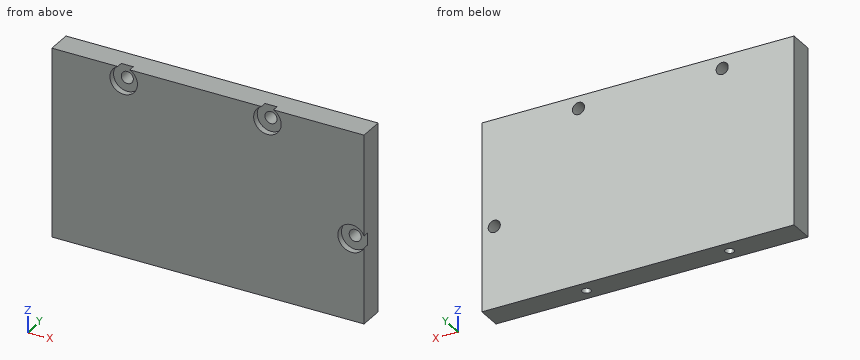
from build123d import *

# Parameters (mm, degrees)
SKETCH1_W                                           = 63
SKETCH1_H                                           = 38
BOSS_EXTRUDE1_DEPTH                                 = 5
CBORE_FOR_2_BINDING_HEAD_MACHINE_SCREW2_D           = 2.4384
CBORE_FOR_2_BINDING_HEAD_MACHINE_SCREW2_CBORE_D     = 5.55752
CBORE_FOR_2_BINDING_HEAD_MACHINE_SCREW2_CBORE_DEPTH = 1.27
CBORE_FOR_2_BINDING_HEAD_MACHINE_SCREW3_D           = 2.4384
CBORE_FOR_2_BINDING_HEAD_MACHINE_SCREW3_CBORE_D     = 5.55752
CBORE_FOR_2_BINDING_HEAD_MACHINE_SCREW3_CBORE_DEPTH = 1.27
F_2_56_TAPPED_HOLE1_D                               = 1.778
F_2_56_TAPPED_HOLE1_DEPTH                           = 9.46583491
F_2_56_TAPPED_HOLE1_TIP                             = 0.53416509


with BuildPart() as part:
    # Sketch1 → Boss-Extrude1 (new body)
    with BuildSketch(Plane(origin=(0, 0, 0), x_dir=(1, 0, 0), z_dir=(0, 1, 0))):
        Rectangle(SKETCH1_W, SKETCH1_H)
    extrude(amount=BOSS_EXTRUDE1_DEPTH)

    # CBORE for #2 Binding Head Machine Screw2 (through all)
    with Locations(Plane(origin=(0, 0, 0), x_dir=(-1, 0, 0), z_dir=(0, -1, 0))):
        with Locations((-29, 2.5)):
            CounterBoreHole(CBORE_FOR_2_BINDING_HEAD_MACHINE_SCREW2_D / 2, CBORE_FOR_2_BINDING_HEAD_MACHINE_SCREW2_CBORE_D / 2, CBORE_FOR_2_BINDING_HEAD_MACHINE_SCREW2_CBORE_DEPTH)

    # CBORE for #2 Binding Head Machine Screw3 (through all)
    with Locations(Plane(origin=(0, 0, 0), x_dir=(-1, 0, 0), z_dir=(0, -1, 0))):
        with Locations((-12, -16.5), (17, -16.5)):
            CounterBoreHole(CBORE_FOR_2_BINDING_HEAD_MACHINE_SCREW3_D / 2, CBORE_FOR_2_BINDING_HEAD_MACHINE_SCREW3_CBORE_D / 2, CBORE_FOR_2_BINDING_HEAD_MACHINE_SCREW3_CBORE_DEPTH)

    # #2-56 Tapped Hole1
    with Locations(Plane(origin=(0, 0, -19), x_dir=(-1, 0, 0), z_dir=(0, 0, -1))):
        with Locations((-11.79093, 2.5), (17.06969, 2.5)):
            Hole(F_2_56_TAPPED_HOLE1_D / 2, depth=F_2_56_TAPPED_HOLE1_DEPTH)
            with Locations((0, 0, -(F_2_56_TAPPED_HOLE1_DEPTH + F_2_56_TAPPED_HOLE1_TIP / 2))):  # 118° drill point
                Cone(0, F_2_56_TAPPED_HOLE1_D / 2, F_2_56_TAPPED_HOLE1_TIP, mode=Mode.SUBTRACT)


solid = part.part
Could you check a few things on this model? Use its own coordinates, in mm. Coordinates: 2 decimals unless noted, no trailing zeros. Write each loop counter-clockwise with the first axis right and the second up, starting at its lowest first coordinate (ties: lowest second). Pieces come first, ordered by that corner, then holes. Notation, with made-up numbers: M 3.5,20.5 L 43.5,20.5 A13 ccw 43.5,33.5 Z; hole C -25,-14.5 d9. An arc over 180 degrees is marked long. One line per question, with ' | ' between items.
1) I need wall thicknesses on probe 1 along X at (y, z) = (0.4, 16.5); probe 2 along X at (y, z) = (2.5, -14.5); probe 3 along Z at (x, y) = (29, 0.4). Which ranges of each line are inside material? Lowest first, please. Write a range as [from, to].
Checks:
probe 1: [-31.5, -19.78], [-14.22, 9.22], [14.78, 31.5] | probe 2: [-31.5, -17.96], [-16.18, 10.9], [12.68, 31.5] | probe 3: [-19, -5.28], [0.28, 19]
2) Imagine slicing it at C-C, the plane z = -14. Write out the boundary of the cut face in (x, y), and give its area (3 significant figures).
Checks:
outline: M -31.5,0 L 31.5,0 L 31.5,5 L -31.5,5 Z; hole C -17.07,2.5 d1.78; hole C 11.79,2.5 d1.78 | area: 310 mm²
3) Imagine slicing it at A-A, the plane z = 16.5. Write out the boundary of the cut face in (x, y).
Checks:
outline: M -31.5,0 L -19.78,0 L -19.78,1.27 L -18.22,1.27 L -18.22,5 L -31.5,5 Z; M -15.78,1.27 L -14.22,1.27 L -14.22,0 L 9.22,0 L 9.22,1.27 L 10.78,1.27 L 10.78,5 L -15.78,5 Z; M 13.22,1.27 L 14.78,1.27 L 14.78,0 L 31.5,0 L 31.5,5 L 13.22,5 Z
4) For pin 1 Ø3.5 at (x, z) = (29, -2.5) entering from -Y, with a flat end and sliding along its axis, tell me the tip position at first contact or that it passes through.
Checks:
pin 1: y = 1.27
5) Imagine slicing it at B-B, the plane z = -2.5. Write out the boundary of the cut face in (x, y).
Checks:
outline: M -31.5,0 L 26.22,0 L 26.22,1.27 L 27.78,1.27 L 27.78,5 L -31.5,5 Z; M 30.22,1.27 L 31.5,1.27 L 31.5,5 L 30.22,5 Z
